from build123d import *

# Parameters (mm, degrees)
SKETCH1_W           = 15
SKETCH1_H           = 15
BOSS_EXTRUDE1_DEPTH = 26
SKETCH2_R           = 1.5
CUT_EXTRUDE1_DEPTH  = 31.939457009
SKETCH3_R           = 7
BOSS_EXTRUDE2_DEPTH = 8
SKETCH4_W           = 10
SKETCH4_H           = 10
BOSS_EXTRUDE3_DEPTH = 7.5
SKETCH5_R           = 5
BOSS_EXTRUDE4_DEPTH = 13
BOSS_EXTRUDE5_START = 5
SKETCH7_R           = 7
BOSS_EXTRUDE5_DEPTH = 5
SKETCH8_W           = 10
SKETCH8_H           = 10
BOSS_EXTRUDE6_DEPTH = 12.5


with BuildPart() as part:
    # Sketch1 → Boss-Extrude1 (new body)
    with BuildSketch(Plane.XY):
        Rectangle(SKETCH1_W, SKETCH1_H)
    extrude(amount=BOSS_EXTRUDE1_DEPTH)

    # Sketch2 → Cut-Extrude1 (cut, through all)
    with BuildSketch(Plane(origin=(0, 7.5, 0), x_dir=(1, 0, 0), z_dir=(0, 1, 0))):
        with Locations(Location((0, -20, 0), (0, 0, 270))):
            Circle(SKETCH2_R)
    extrude(amount=-CUT_EXTRUDE1_DEPTH, mode=Mode.SUBTRACT)

    # Sketch3 → Boss-Extrude2 (add)
    with BuildSketch(Plane.XY.offset(26)):
        Circle(SKETCH3_R)
    extrude(amount=BOSS_EXTRUDE2_DEPTH)

    # Sketch4 → Boss-Extrude3 (add)
    with BuildSketch(Plane.XY.offset(34)):
        Rectangle(SKETCH4_W, SKETCH4_H)
    extrude(amount=BOSS_EXTRUDE3_DEPTH)

    # Sketch5 → Boss-Extrude4 (add)
    with BuildSketch(Plane.XY.offset(41.5)):
        Circle(SKETCH5_R)
    extrude(amount=BOSS_EXTRUDE4_DEPTH)

    # Sketch6 → Revolve1 (revolve)
    with BuildSketch(Plane(origin=(0, 0, 0), x_dir=(1, 0, 0), z_dir=(0, 1, 0)), mode=Mode.PRIVATE) as revolve1_sk:
        with BuildLine():
            Line((0, -54.5), (5, -54.5))
            ThreePointArc((5, -54.5), (2.582569334, -55.466460537), (0, -55.795630141))
            Line((0, -55.795630141), (0, -54.5))
        make_face()
    revolve(revolve1_sk.sketch.rotate(Axis((0, 0, 54.5), (0, 0, 1)), 224.415308597), axis=Axis((0, 0, 54.5), (0, 0, 1)))

    # Sketch7 → Boss-Extrude5 (add)
    with BuildSketch(Plane(origin=(0, 0, 0), x_dir=(-1, 0, 0), z_dir=(0, 0, -1)).offset(BOSS_EXTRUDE5_START)):
        with Locations(Location((0, 0, 0), (0, 0, 315.584691403))):
            Circle(SKETCH7_R)
    extrude(amount=-BOSS_EXTRUDE5_DEPTH)

    # Sketch8 → Boss-Extrude6 (add)
    with BuildSketch(Plane(origin=(0, 0, -5), x_dir=(-1, 0, 0), z_dir=(0, 0, -1))):
        Rectangle(SKETCH8_W, SKETCH8_H)
    extrude(amount=BOSS_EXTRUDE6_DEPTH)


solid = part.part
CAD build for the part. Positions are in the model's coordinates, mm. A direction names the side the tool comes from. Round coordinates to 2 decimals unless told otherwise and drop trailing zeros. Order: outer loops, then holes, each group sorted by start corner. A loop starts at its lowest first (then second) coordinate and runs counter-clockwise, first axis right, second up. Notation, with made-up numbers: (47.25, 71.5) -> (74.25, 71.5) arc R32 cw to (74.25, 110.5) -> close; hole circle Ø7 at (-31.5, -37.5). An arc over 180 degrees is marked (long way). Write item = value, one per line. Start each with the question number.
(1) Cut at B-B, the plane y = 6. List the corners of the cut face in (x, z).
(2) Pin check, flat tips, straight feed: P1, Ø4, axis at x = -2, y = 2.5, coming from the +Z side; P2, Ø4, axis at x = 2.5, y = 1.5, coming from the +Z side; P3, Ø2, axis at y = -2, z = 36.5, coming from the +X side; P4, Ø2.5, axis at x = 0, z = 20, coming from the +Y side. Stop position of each tip, or through.
(3) Cut at D-D, the plane z = 45.5. List the corners of the cut face in (x, y), then the cut area to 3 significant figures.
(4) Cut at C-C, the plane x = -4.25. List the corners of the cut face in (y, z) (1 decimal), then the cut area to 3 significant figures.
(5) Probe line 1 (X direction, y = -1.25, z = 20); line 2 (Y direction, x = -3.5, z = -10); line 3 (Z direction, x = -3.25, y = 4). List the from-to ranges inside material, lowest first. Write a range as [from, to].
(6) Which spindle directions (+Z, -Z, +X, -X, +Y, -Y) get a long thin tool onto all of the face, cutting with end or side? Do faces 1 (the flat face through (0, -5, -11)), 2 (the flat face through (6, 0, 34)), 3 (the flat face through (4, -4, 41.5)), 4 (the flat face through (0, 5, -11)), 5 (the flat face through (-6, 0, -5)). Say none if no direction does.
(7) Cut at A-A, the plane z = 20. List the corners of the cut face in (x, y), then the cut area to 3 significant figures.
Model answer:
q1.outline = (-7.5, 0) -> (-3.61, 0) -> (-3.61, -5) -> (3.61, -5) -> (3.61, 0) -> (7.5, 0) -> (7.5, 26) -> (3.61, 26) -> (3.61, 34) -> (-3.61, 34) -> (-3.61, 26) -> (-7.5, 26) -> close; hole circle Ø3 at (0, 20)
q2.P1 = 55.73
q2.P2 = 55.75
q2.P3 = 5
q2.P4 = through
q3.outline = circle Ø10 at (0, 0)
q3.area = 78.5 mm2
q4.outline = (-7.5, 0) -> (-5.6, 0) -> (-5.6, -5) -> (-5, -5) -> (-5, -17.5) -> (5, -17.5) -> (5, -5) -> (5.6, -5) -> (5.6, 0) -> (7.5, 0) -> (7.5, 26) -> (5.6, 26) -> (5.6, 34) -> (5, 34) -> (5, 41.5) -> (2.6, 41.5) -> (2.6, 54.5) arc R9.4 ccw to (-2.6, 54.5) -> (-2.6, 41.5) -> (-5, 41.5) -> (-5, 34) -> (-5.6, 34) -> (-5.6, 26) -> (-7.5, 26) -> close
q4.area = 804 mm2
q5.line_1 = [-7.5, -1.5], [1.5, 7.5]
q5.line_2 = [-5, 5]
q5.line_3 = [-17.5, 41.5]
q6.face_1 = -Z, +X, -X, -Y
q6.face_2 = +Z, +X, +Y, -Y
q6.face_3 = +Z, +X, -Y
q6.face_4 = -Z, +X, -X, +Y
q6.face_5 = -Z, -X, +Y, -Y
q7.outline = (-7.5, -7.5) -> (-1.5, -7.5) -> (-1.5, 7.5) -> (-7.5, 7.5) -> close; (1.5, -7.5) -> (7.5, -7.5) -> (7.5, 7.5) -> (1.5, 7.5) -> close
q7.area = 180 mm2
